```python
from build123d import *

# Parameters (mm, degrees)
SKETCH1_W           = 20
SKETCH1_H           = 20
SKETCH1_R           = 4.683092763
BOSS_EXTRUDE1_DEPTH = 100
SKETCH2_R           = 2.5
CUT_EXTRUDE1_DEPTH  = 100
SKETCH3_R           = 2.5
CUT_EXTRUDE2_DEPTH  = 103.469507777


with BuildPart() as part:
    # Sketch1 → Boss-Extrude1 (new body)
    with BuildSketch(Plane(origin=(0, 0, 0), x_dir=(1, 0, 0), z_dir=(0, 1, 0))):
        Rectangle(SKETCH1_W, SKETCH1_H)
        with Locations(Location((0, 0, 0), (0, 0, 270))):
            Circle(SKETCH1_R, mode=Mode.SUBTRACT)
    extrude(amount=BOSS_EXTRUDE1_DEPTH)

    # Sketch2 → Cut-Extrude1 (cut)
    with BuildSketch(Plane.XY.offset(10)):
        with Locations((0, 5)):
            Circle(SKETCH2_R)
    extrude(amount=-CUT_EXTRUDE1_DEPTH, mode=Mode.SUBTRACT)

    # Sketch3 → Cut-Extrude2 (cut, through all)
    with BuildSketch(Plane.XY.offset(10)):
        with Locations((0, 60)):
            Circle(SKETCH3_R)
        with Locations((0, 70)):
            Circle(SKETCH3_R)
    extrude(amount=-CUT_EXTRUDE2_DEPTH, mode=Mode.SUBTRACT)


solid = part.part
```
Source: CAD feature listing. Evaluate the final solid. Frame: model axes, mm. Give positions to 0.01 mm unless a question says otherwise; leave off trailing zeros. Write each loop counter-clockwise with the first axis right and the second up, starting at its lowest first coordinate (ties: lowest second). Pieces come first, ordered by that corner, then holes. Notation, with made-up numbers: (22, 37.5) - (74, 37.5) arc R4 cw to (74, 42.5) - close; hole circle Ø11 at (19.5, 56.5). An arc over 180 degrees is marked (long way). One line per item, written item: value. Start each with the question number.
Q1. Section query C-C, the plane x = 0. Count the separate pieces of the cut face and the enclosed holes in it, then the cut area to 3 significant figures.
Q2. Section query A-A, the plane z = 0. Return the cut outline in (x, y), then the cut area to 3 significant figures.
Q3. Section query D-D, the plane z = -7. Return the cut outline in (x, y), then the cut area to 3 significant figures.
Q4. Section query B-B, the plane y = 60. Return the cut outline in (x, z), then the cut area to 3 significant figures.
Q5. Material intervals for probe 1 along Y at (x, z) = (0, -8.5); probe 2 along X at (y, z) = (60, 8.75); probe 3 along X at (y, z) = (16.5, -1), sorted ascending. Write a range as from..to.
Q6. Draft query along Y for faces 1 (the face through (-2.5, 60.1, 7)), 2 (the face through (-2.5, 70.1, 7)), 3 (the face through (0, 49, -10)), 4 (the face through (-2, 0, -5)). Return one class per face: +Y half, -Y half, draft (parallel to the pull), parting line (faces both ways), or undercut.
Q7. First-contact query: pin 1 Ø4.5 at (x, y) = (0, 5) entering from +Z. Flat tip, straight axial feed; report the tip coordinate or a pass-through.
Answer:
1. separate pieces: 8
1. enclosed holes: 0
1. area: 904 mm2
2. outline: (-10, 0) - (-4.68, 0) - (-4.68, 100) - (-10, 100) - close; (4.68, 0) - (10, 0) - (10, 100) - (4.68, 100) - close
2. area: 1,060 mm2
3. outline: (-10, 0) - (10, 0) - (10, 100) - (-10, 100) - close; hole circle Ø5 at (0, 5); hole circle Ø5 at (0, 60); hole circle Ø5 at (0, 70)
3. area: 1,940 mm2
4. outline: (-10, -10) - (-2.5, -10) - (-2.5, -3.96) arc R4.68 cw to (-2.5, 3.96) - (-2.5, 10) - (-10, 10) - close; (2.5, -10) - (10, -10) - (10, 10) - (2.5, 10) - (2.5, 3.96) arc R4.68 cw to (2.5, -3.96) - close
4. area: 276 mm2
5. probe 1: y = 0..2.5, 7.5..57.5, 62.5..67.5, 72.5..100
5. probe 2: x = -10..-2.5, 2.5..10
5. probe 3: x = -10..-4.58, 4.58..10
6. face 1: undercut
6. face 2: undercut
6. face 3: draft
6. face 4: -Y half
7. pin 1: passes through
